Can you work these out from the model? Positions are in its coordinate system, mm. Face numbers are marked on the shaded views. A direction names the side the tool comes from. Coordinates: 2 decimals unless noted, no trailing zeros. Loops run counter-clockwise (first coordinate to the right, second up) from the corner with the lowest first, then second, coordinate; pieces in that order, holes last.
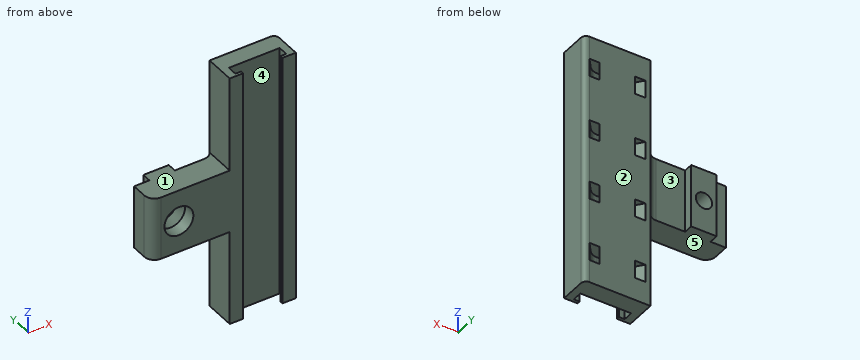
```python
from build123d import *

# Parameters (mm, degrees)
PAD009_DEPTH    = 12.5
POCKET001_DEPTH = 1.75
PAD013_DEPTH    = 12.5


with BuildPart() as f_12_5mm_segment:
    # Sketch015 → Pad009 (new body)
    with BuildSketch(Plane.XY):
        with BuildLine():
            Line((10, -9), (10, -15))
            Line((10, -15), (12.625, -15))
            Line((12.625, -15), (12.625, -14.4))
            Line((12.625, -14.4), (11.5, -14.4))
            Line((11.5, -14.4), (11.5, -12.45))
            Line((11.5, -12.45), (21.5, -12.45))
            Line((21.5, -12.45), (21.5, -14.4))
            Line((21.5, -14.4), (20.375, -14.4))
            Line((20.375, -14.4), (20.375, -15))
            Line((20.375, -15), (23, -15))
            Line((23, -15), (23, -10))
            ThreePointArc((23, -10), (22.707107, -9.292893), (22, -9))
            Line((22, -9), (10, -9))
        make_face()
    extrude(amount=PAD009_DEPTH)

    # Sketch016 → Pocket001 (cut, symmetric)
    with BuildSketch(Plane(origin=(0, 0, 6.25), x_dir=(1, 0, 0), z_dir=(0, 0, -1))):
        with BuildLine():
            ThreePointArc((14.83303, 10.2), (13.737585, 9.87332), (13, 9))
            Line((11, 9), (13, 9))
            Line((12.497007, 10.860502), (11, 9))
            ThreePointArc((14.25, 11.7), (13.27818, 11.479302), (12.497007, 10.860502))
            Line((14.25, 11.7), (18.75, 11.7))
            ThreePointArc((20.502993, 10.860502), (19.72182, 11.479302), (18.75, 11.7))
            Line((20.502993, 10.860502), (22, 9))
            Line((22, 9), (20, 9))
            ThreePointArc((20, 9), (19.262415, 9.87332), (18.16697, 10.2))
            Line((14.83303, 10.2), (18.16697, 10.2))
        make_face()
    extrude(amount=POCKET001_DEPTH, both=True, mode=Mode.SUBTRACT)


with BuildPart() as obj1:
    # Body019 base: copy of 12.5mm-Segment
    add(f_12_5mm_segment.part)


with BuildPart() as obj2:
    # Body022 base: copy of obj1
    add(obj1.part)


with BuildPart() as obj2_1:
    # Body022 placement: moved
    add(obj2.part.moved(Location((0, 0, 12.5))))


with BuildPart() as obj3:
    # Body012004 base: copy of 12.5mm-Segment
    add(f_12_5mm_segment.part)


with BuildPart() as obj3_1:
    # Body012004 placement: moved
    add(obj3.part.moved(Location((0, 0, 25))))


with BuildPart() as obj4:
    # Body012005 base: copy of 12.5mm-Segment
    add(f_12_5mm_segment.part)


with BuildPart() as obj4_1:
    # Body012005 placement: moved
    add(obj4.part.moved(Location((0, 0, 37.5))))


with BuildPart() as obj5:
    # Sketch027 → Pad013 (new body)
    with BuildSketch(Plane.XY):
        with BuildLine():
            Line((-3.5, -15), (10, -15))
            Line((10, -9), (10, -15))
            ThreePointArc((8.267949, -10), (9.267949, -9.732051), (10, -9))
            Line((2.5, -10), (8.267949, -10))
            Line((2.5, -8.2), (2.5, -10))
            Line((-2.5, -8.2), (2.5, -8.2))
            Line((-2.5, -10), (-2.5, -8.2))
            Line((-5.5, -10), (-2.5, -10))
            Line((-5.5, -13), (-5.5, -10))
            ThreePointArc((-5.5, -13), (-4.914214, -14.414214), (-3.5, -15))
        make_face()
    extrude(amount=PAD013_DEPTH)

    # Sketch028 → Groove (revolve, cut)
    with BuildSketch(Plane(origin=(0, -11, 6.25), x_dir=(-1, 0, 0), z_dir=(0, 0, 1))):
        Polygon((0, 4), (2.85, 4), (2.85, 1.5), (1.6, 0.25), (1.6, -7.75), (0, -7.75), align=None)
    revolve(axis=Axis((0, -11, 6.25), (0, -1, 0)), mode=Mode.SUBTRACT)


with BuildPart() as obj5_1:
    # Body018 placement: moved
    add(obj5.part.moved(Location((0, 0, 18.75))))

    # Fusion: union obj1, obj2, obj3, obj4
    add(obj1.part)
    add(obj2_1.part)
    add(obj3_1.part)
    add(obj4_1.part)


with BuildPart() as obj5_2:
    # Fusion placement: moved
    add(obj5_1.part.moved(Location((0, 0, 10))))


solid = obj5_2.part
```
Item 1: Suppose I cut it at C-C, the plane z = 56. Please give me the cut outline in (x, y) (3 decimals).
Results are:
outline: (10, -15) - (12.625, -15) - (12.625, -14.4) - (11.5, -14.4) - (11.5, -12.45) - (21.5, -12.45) - (21.5, -14.4) - (20.375, -14.4) - (20.375, -15) - (23, -15) - (23, -10) arc R1 ccw to (22, -9) - (10, -9) - close
Item 2: Suppose I cut it at D-D, the plane x = 6. Please give me the cut outline in (y, z), plus the area to 3 significant figures.
Results are:
outline: (-15, 28.75) - (-10, 28.75) - (-10, 41.25) - (-15, 41.25) - close
area: 62.5 mm2
Item 3: I need wall thicknesses on line 1 along X through (y, z) = (-13.2, 35); line 2 along Z through (x, y) = (12.5, -10); line 3 along Z through (x, y) = (0, -13.9). Which ranges of each line are inside material? Lowest first, please.
Results are:
line 1: x = -5.49 to -2.85, 2.85 to 11.5, 21.5 to 23
line 2: z = 10 to 14.5, 18 to 27, 30.5 to 39.5, 43 to 52, 55.5 to 60
line 3: z = 28.75 to 32.15, 37.85 to 41.25
Item 4: On a 3-axis mill with a long thin cutter (end or side, diameter ignored), from which of +Z, -Z, +X, -X, +Y, -Y can I reach the whole of each face in a straight line? I mean the marked faces 1, 2, 3, 4 and 5. Say none if no direction works.
Results are:
face 1: +Z, -X, +Y, -Y
face 2: +Z, -Z, +X, +Y
face 3: +Z, -Z, +Y
face 4: +Z, -Z
face 5: -Z, -X, +Y, -Y
Item 5: I'm going to push flat-ended pins straight in: P1, Ø3.5, axis at x = 16.5, z = 16, coming from the -Y side; P2, Ø2, axis at y = -8.5, z = 35.5, coming from the +X side; P3, Ø6, axis at x = 13, z = 50, coming from the -Y side; P4, Ø8, axis at x = 19, z = 21.5, coming from the +Y side. Where does each tip first touch, or does it pass through?
Results are:
P1: stops at y = -12.45
P2: stops at x = 22.87
P3: stops at y = -15
P4: stops at y = -9
Item 6: Suppose I cut it at A-A, the plane x = 0. Please give me the cut outline in (y, z), plus the area to 3 significant figures.
Results are:
outline: (-15, 28.75) - (-8.2, 28.75) - (-8.2, 33.4) - (-11.25, 33.4) - (-12.5, 32.15) - (-15, 32.15) - close; (-15, 37.85) - (-12.5, 37.85) - (-11.25, 36.6) - (-8.2, 36.6) - (-8.2, 41.25) - (-15, 41.25) - close
area: 55.4 mm2
